The listing builds one solid part. Answer for the finished solid, in the listing's coordinates (mm). A direction names the side the tool comes from. Round coordinates to 2 decimals unless told otherwise and drop trailing zeros. Write each loop counter-clockwise with the first axis right and the second up, starting at its lowest first coordinate (ties: lowest second). Pieces come first, ordered by that corner, then holes. Notation, with made-up numbers: (49, 0.5) - (78, 0.5) arc R22 ccw to (78, 9.5) - close; hole circle Ø2 at (18.25, -27.5). An arc over 180 degrees is marked (long way). Answer in a Markdown table with one row per item.
from build123d import *

# Parameters (mm, degrees)
SKETCH1_R           = 2.5
BOSS_EXTRUDE1_DEPTH = 10
SKETCH2_W           = 120
SKETCH2_H           = 60
SKETCH2_R           = 2.5
BOSS_EXTRUDE2_DEPTH = 10
BOSS_EXTRUDE3_DEPTH = 10


with BuildPart() as part:
    # Sketch1 → Boss-Extrude1 (new body)
    with BuildSketch(Plane.XY):
        Polygon((-29.5, 25), (-29.5, 35), (29.5, 35), (29.5, 25), (29.5, -25), (-29.5, -25), align=None)
        with Locations((-20, 15)):
            Circle(SKETCH1_R, mode=Mode.SUBTRACT)
        with Locations((20, 15)):
            Circle(SKETCH1_R, mode=Mode.SUBTRACT)
        with Locations((20, -15)):
            Circle(SKETCH1_R, mode=Mode.SUBTRACT)
        with Locations((-20, -15)):
            Circle(SKETCH1_R, mode=Mode.SUBTRACT)
    extrude(amount=BOSS_EXTRUDE1_DEPTH)

    # Sketch2 → Boss-Extrude2 (add)
    with BuildSketch(Plane(origin=(0, 35, 0), x_dir=(1, 0, 0), z_dir=(0, 1, 0))):
        with Locations((0, -40)):
            Rectangle(SKETCH2_W, SKETCH2_H)
        with Locations((20, -25)):
            Circle(SKETCH2_R, mode=Mode.SUBTRACT)
        with Locations((35, -35)):
            Circle(SKETCH2_R, mode=Mode.SUBTRACT)
        with BuildLine():
            Line((-55, -37.5), (-20, -37.5))
            ThreePointArc((-20, -37.5), (-17.5, -40), (-20, -42.5))
            Line((-20, -42.5), (-55, -42.5))
            ThreePointArc((-55, -42.5), (-57.5, -40), (-55, -37.5))
        make_face(mode=Mode.SUBTRACT)
        with BuildLine():
            Line((-2.5, -65), (-2.5, -50))
            ThreePointArc((-2.5, -50), (0, -47.5), (2.5, -50))
            Line((2.5, -50), (2.5, -65))
            ThreePointArc((2.5, -65), (0, -67.5), (-2.5, -65))
        make_face(mode=Mode.SUBTRACT)
    extrude(amount=-BOSS_EXTRUDE2_DEPTH)

    # Sketch4 → Boss-Extrude3 (add)
    with BuildSketch(Plane(origin=(14.5, 0, 0), x_dir=(0, 0, -1), z_dir=(1, 0, 0))):
        Polygon((-40, 25), (-10, 25), (-10, -5), align=None)
    boss_extrude3 = extrude(amount=-BOSS_EXTRUDE3_DEPTH)

    # Mirror1: Boss-Extrude3 across plane
    add(boss_extrude3.mirror(Plane(origin=(0, 0, 0), x_dir=(0, 0, 1), z_dir=(1, 0, 0))))


solid = part.part
(1) Flat-ended cylindrical pins translate along their axes: pin 1 (12 mm diameter, centred on x = -19.5, y = 7, fed in from +Z); pin 2 (12 mm diameter, centred on y = 20.5, z = 61.5, fed in from +X); pin 3 (4.5 mm diameter, centred on x = 20, z = 25, fed in from -Y); pin 4 (5 mm diameter, centred on x = -43.5, y = 28.5, fed in from -Z). Find the tip coordinate at first contact, or state that the pin passes through.
Checked values:
| item | result |
|---|---|
| pin 1 | stops at z = 25.32 |
| pin 2 | stops at x = 60 |
| pin 3 | passes through |
| pin 4 | stops at z = 10 |
(2) Section C-C (y = -15) is taken. Give the vertices of the cut face in (x, z), and give its area (3 significant figures).
Checked values:
| item | result |
|---|---|
| outline | (-29.5, 0) - (-22.5, 0) - (-22.5, 10) - (-29.5, 10) - close; (-17.5, 0) - (17.5, 0) - (17.5, 10) - (-17.5, 10) - close; (22.5, 0) - (29.5, 0) - (29.5, 10) - (22.5, 10) - close |
| area | 490 mm2 |
(3) For faces 4 (the flat face through (-29.5, 5, 5)), 5 (the flat face through (-14.5, 14, 21)), 6 (the flat face through (2.5, 30, 57)), 7 (the flat face through (4.5, 14, 21)), 8 (the flat face through (14.5, 14, 21)), determine the directions among +Z, -Z, +X, -X, +Y, -Y from which every point of the face is accessible in a straight line to the end or side of a thin tool.
Checked values:
| item | result |
|---|---|
| face 4 | -Z, -X, +Y, -Y |
| face 5 | +Z, -X, -Y |
| face 6 | +Y, -Y |
| face 7 | +Z, -Y |
| face 8 | +Z, +X, -Y |
(4) Find the intervals of material crossed by line 1 (Z direction, x = 20, y = 30.25); line 2 (Y direction, x = 20, z = 5.75); line 3 (X direction, y = 29.25, z = 35), in increasing order.
Checked values:
| item | result |
|---|---|
| line 1 | z = 0 to 22.5, 27.5 to 70 |
| line 2 | y = -25 to -17.5, -12.5 to 12.5, 17.5 to 35 |
| line 3 | x = -60 to 32.5, 37.5 to 60 |
(5) Section D-D (x = 20) is taken. Give the vertices of the cut face in (y, z).
Checked values:
| item | result |
|---|---|
| outline | (-25, 0) - (-17.5, 0) - (-17.5, 10) - (-25, 10) - close; (-12.5, 0) - (12.5, 0) - (12.5, 10) - (-12.5, 10) - close; (17.5, 0) - (35, 0) - (35, 22.5) - (25, 22.5) - (25, 10) - (17.5, 10) - close; (25, 27.5) - (35, 27.5) - (35, 70) - (25, 70) - close |
(6) For a pull along Y with two mould halves and no side action, classify faces 1 (the cylindrical face through (-0.1, 30.1, 47.5)), 2 (the cylindrical face through (17.5, 15.1, 4.9)), 3 (the flat face through (0, -25, 5)) as pulls with the +Y half, pulls with the -Y half, needs draft (parallel to the pull), parting line crosses it, or undercut.
Checked values:
| item | result |
|---|---|
| face 1 | needs draft |
| face 2 | undercut |
| face 3 | pulls with the -Y half |
(7) Section A-A (z = 61) is taken. Give the vertices of the cut face in (x, y), and give its area (3 significant figures).
Checked values:
| item | result |
|---|---|
| outline | (-60, 25) - (-2.5, 25) - (-2.5, 35) - (-60, 35) - close; (2.5, 25) - (60, 25) - (60, 35) - (2.5, 35) - close |
| area | 1,150 mm2 |
(8) Section B-B (x = -34.5) is taken. Give the vertices of the cut face in (y, z), and give its area (3 significant figures).
Checked values:
| item | result |
|---|---|
| outline | (25, 10) - (35, 10) - (35, 37.5) - (25, 37.5) - close; (25, 42.5) - (35, 42.5) - (35, 70) - (25, 70) - close |
| area | 550 mm2 |
